Design review of the part built by this model. Coordinates are the model's own, in mm. A direction names the side the tool comes from. Give positions to 0.01 mm unless a question says otherwise; leave off trailing zeros. Loops run counter-clockwise (first coordinate to the right, second up) from the corner with the lowest first, then second, coordinate; pieces in that order, holes last.
from build123d import *

# Parameters (mm, degrees)
SKIZZE1_W                       = 250
SKIZZE1_H                       = 125
AUFSATZ_LINEAR_AUSTRAGEN1_DEPTH = 2
SKIZZE2_W                       = 100
SKIZZE2_H                       = 100
AUFSATZ_LINEAR_AUSTRAGEN2_DEPTH = 100
SCHNITT_LINEAR_AUSTRAGEN1_DEPTH = 100
SCHNITT_LINEAR_AUSTRAGEN2_DEPTH = 100
SKIZZE6_W                       = 242
SKIZZE6_H                       = 117
AUFSATZ_LINEAR_AUSTRAGEN3_DEPTH = 2
SKIZZE7_R                       = 2
SCHNITT_LINEAR_AUSTRAGEN5_DEPTH = 32


with BuildPart() as part:
    # Skizze1 → Aufsatz-Linear austragen1 (new body)
    with BuildSketch(Plane.XY):
        with Locations((125, 62.5)):
            Rectangle(SKIZZE1_W, SKIZZE1_H)
    extrude(amount=AUFSATZ_LINEAR_AUSTRAGEN1_DEPTH)

    # Skizze2 → Aufsatz-Linear austragen2 (add)
    with BuildSketch(Plane.XY.offset(2)):
        with Locations((125, 75)):
            Rectangle(SKIZZE2_W, SKIZZE2_H)
    extrude(amount=AUFSATZ_LINEAR_AUSTRAGEN2_DEPTH)

    # Skizze3 → Schnitt-Linear austragen1 (cut)
    with BuildSketch(Plane.ZY.offset(-75)):
        Polygon((102, 25), (102, 125), (2, 125), align=None)
    extrude(amount=-SCHNITT_LINEAR_AUSTRAGEN1_DEPTH, mode=Mode.SUBTRACT)

    # Skizze4 → Schnitt-Linear austragen2 (cut)
    with BuildSketch(Plane.ZY.offset(-75)):
        Polygon((2, 119.343145751), (92.343145751, 29), (2, 29), align=None)
    extrude(amount=-SCHNITT_LINEAR_AUSTRAGEN2_DEPTH, mode=Mode.SUBTRACT)

    # Skizze6 → Aufsatz-Linear austragen3 (add)
    with BuildSketch(Plane(origin=(0, 0, 0), x_dir=(-1, 0, 0), z_dir=(0, 0, -1))):
        with Locations((-125, 62.5)):
            Rectangle(SKIZZE6_W, SKIZZE6_H)
    extrude(amount=AUFSATZ_LINEAR_AUSTRAGEN3_DEPTH)

    # Skizze7 → Schnitt-Linear austragen5 (cut)
    with BuildSketch(Plane(origin=(0, 0, -2), x_dir=(-1, 0, 0), z_dir=(0, 0, -1))):
        with Locations((-243, 118)):
            Circle(SKIZZE7_R)
        with Locations((-7, 7)):
            Circle(SKIZZE7_R)
        with Locations((-7, 118)):
            Circle(SKIZZE7_R)
        with Locations((-243, 7)):
            Circle(SKIZZE7_R)
    extrude(amount=-SCHNITT_LINEAR_AUSTRAGEN5_DEPTH, mode=Mode.SUBTRACT)


solid = part.part
Q1. Take a section at B-B (z = 77.5). Give the boundary of the cut face in (x, y), plus the area to 3 significant figures.
Results:
outline: (75, 25) - (175, 25) - (175, 29) - (75, 29) - close; (75, 43.84) - (175, 43.84) - (175, 49.5) - (75, 49.5) - close
area: 966 mm2
Q2. Take a section at A-A (x = 149.5). Give the boundary of the cut face in (y, z), plus the area to 3 significant figures.
Results:
outline: (0, 0) - (4, 0) - (4, -2) - (121, -2) - (121, 0) - (125, 0) - (125, 2) - (25, 102) - (25, 2) - (0, 2) - close; hole (29, 2) - (119.34, 2) - (29, 92.34) - close
area: 1,400 mm2
Q3. Take a section at C-C (y = 76.5). Give the boundary of the cut face in (x, z).
Results:
outline: (0, 0) - (4, 0) - (4, -2) - (246, -2) - (246, 0) - (250, 0) - (250, 2) - (0, 2) - close; (75, 44.84) - (175, 44.84) - (175, 50.5) - (75, 50.5) - close
Q4. Draft analysis for pull direction X (two halves, no side actions). For faces 3 (the face through (175, 67, 55)), 4 (the face through (75, 67, 55)), 5 (the face through (124, 25, 51)), state which applies: pulls with the +X half, pulls with the -X half, needs draft (parallel to the pull), parting line crosses it, or undercut.
Results:
face 3: pulls with the +X half
face 4: pulls with the -X half
face 5: needs draft
Q5. Tool access review of faces 1 (the face through (124, 76, 51)), 2 (the face through (124.3, 74.804, 46.539)): name each direction out of +Z, -Z, +X, -X, +Y, -Y from which nothing blocks a thin tool from reaching the whole face with its end or side.
Results:
face 1: +Z, +X, -X, +Y
face 2: +X, -X
Q6. Take a section at D-D (x = 57.5). Give the boundary of the cut face in (y, z).
Results:
outline: (0, 0) - (4, 0) - (4, -2) - (121, -2) - (121, 0) - (125, 0) - (125, 2) - (0, 2) - close
Q7. Insertion check: pin 1 (4.5 mm diameter, centred on x = 243, y = 7, fed in from +Z); pin 2 (4 mm diameter, centred on x = 111, z = 27.5, fed in from +Y); pin 3 (0.6 mm diameter, centred on y = 67.5, z = -1, fed in from +X). Each pin has a flat end and moves straight along its axis. Give the tip position at first contact, or say it passes through.
Results:
pin 1: stops at z = 2
pin 2: stops at y = 101.5
pin 3: stops at x = 246
Q8. Wall thickness on line 1 (Y direction, x = 243, z = -0.2); line 2 (Y direction, x = 7, z = 0.95); line 3 (Z direction, x = 191, y = 65.5): over which ranges is each line inside the solid? List them lowest first.
Results:
line 1: y = 4 to 5, 9 to 116, 120 to 121
line 2: y = 0 to 5, 9 to 116, 120 to 125
line 3: z = -2 to 2
